Read the model definition and answer for the solid it produces. Units are mm, in the model's axes. Coordinates: 2 decimals unless noted, no trailing zeros. Loops run counter-clockwise (first coordinate to the right, second up) from the corner with the lowest first, then second, coordinate; pieces in that order, holes last.
Q1. Straight lines are drawn through the part: line 1 (X direction, y = 5.1, z = 127.5); line 2 (X direction, y = 0.55, z = 251); line 3 (Y direction, x = 12, z = 236.5). For each, find the intervals that lie inside material, in ascending order.
Q2. Section A-A (z = 50) is taken. Give the vertices of the cut face in (x, y), then the cut area to 3 significant figures.
Q3. Section B-B (y = 3.65) is taken. Give the vertices of the cut face in (x, z).
Q4. Flat-ended cylindrical pins translate along their axes: P1, Ø1.5, axis at y = 2.5, z = 259.5, coming from the +X side; P2, Ø1.1, axis at x = -19, y = 0.5, coming from the +Z side; P3, Ø4, axis at x = -20.5, z = 234.5, coming from the +Y side. Find the tip coordinate at first contact, or state that the pin passes through.
Q5. Section C-C (x = 2) is taken. Count the separate pieces of the cut face and the enclosed holes in it, then the cut area to 3 significant figures.
from build123d import *

# Parameters (mm, degrees)
BOSS_EXTRUDE1_DEPTH   = 320
BOSS_EXTRUDE1_2_DEPTH = 320
SKETCH3_W             = 45
SKETCH3_H             = 6
BOSS_EXTRUDE2_DEPTH   = 1


with BuildPart() as part:
    # Sketch1 → Boss-Extrude1 (new body)
    with BuildSketch(Plane.XY):
        Polygon((-17.5, 0), (-17.5, 6), (-15.5, 6), (-15.5, 1), (-11.5, 1), (-11.5, 0), align=None)
    extrude(amount=BOSS_EXTRUDE1_DEPTH)



with BuildPart() as body_2:
    # Sketch1 → Boss-Extrude1 2 (new body)
    with BuildSketch(Plane.XY):
        Polygon((17.5, 0), (17.5, 6), (15.5, 6), (15.5, 1), (11.5, 1), (11.5, 0), align=None)
    extrude(amount=BOSS_EXTRUDE1_2_DEPTH)


with BuildPart() as part_1:
    add(part.part)

    add(body_2.part)  # Boss-Extrude2 merges body 2
    # Sketch3 → Boss-Extrude2 (add)
    with BuildSketch(Plane(origin=(0, 0, 0), x_dir=(1, 0, 0), z_dir=(0, 1, 0))):
        with Locations((0, -14)):
            Rectangle(SKETCH3_W, SKETCH3_H)
        with Locations((0, -36)):
            Rectangle(SKETCH3_W, SKETCH3_H)
        with Locations((0, -58)):
            Rectangle(SKETCH3_W, SKETCH3_H)
        with Locations((0, -80)):
            Rectangle(SKETCH3_W, SKETCH3_H)
        with Locations((0, -102)):
            Rectangle(SKETCH3_W, SKETCH3_H)
        with Locations((0, -124)):
            Rectangle(SKETCH3_W, SKETCH3_H)
        with Locations((0, -146)):
            Rectangle(SKETCH3_W, SKETCH3_H)
        with Locations((0, -168)):
            Rectangle(SKETCH3_W, SKETCH3_H)
        with Locations((0, -190)):
            Rectangle(SKETCH3_W, SKETCH3_H)
        with Locations((0, -212)):
            Rectangle(SKETCH3_W, SKETCH3_H)
        with Locations((0, -234)):
            Rectangle(SKETCH3_W, SKETCH3_H)
        with Locations((0, -256)):
            Rectangle(SKETCH3_W, SKETCH3_H)
        with Locations((0, -278)):
            Rectangle(SKETCH3_W, SKETCH3_H)
        with Locations((0, -300)):
            Rectangle(SKETCH3_W, SKETCH3_H)
    extrude(amount=BOSS_EXTRUDE2_DEPTH)


solid = part_1.part
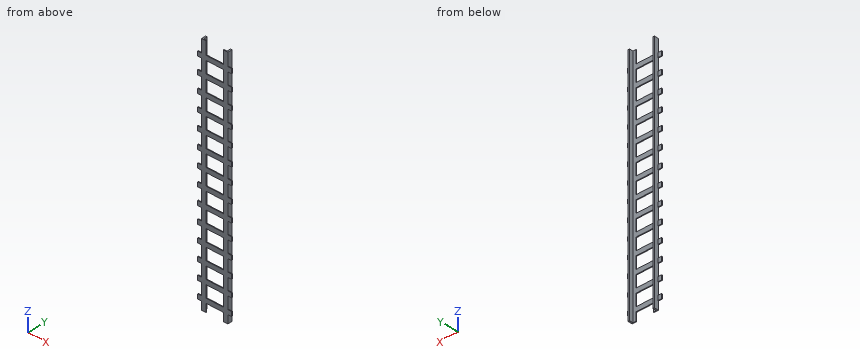
Numbers:
1. line 1: x = -17.5 to -15.5, 15.5 to 17.5
1. line 2: x = -17.5 to -11.5, 11.5 to 17.5
1. line 3: y = 0 to 1
2. outline: (-17.5, 0) - (-11.5, 0) - (-11.5, 1) - (-15.5, 1) - (-15.5, 6) - (-17.5, 6) - close; (11.5, 0) - (17.5, 0) - (17.5, 6) - (15.5, 6) - (15.5, 1) - (11.5, 1) - close
2. area: 32.0 mm2
3. outline: (-17.5, 0) - (-15.5, 0) - (-15.5, 320) - (-17.5, 320) - close; (15.5, 0) - (17.5, 0) - (17.5, 320) - (15.5, 320) - close
4. P1: stops at x = 17.5
4. P2: stops at z = 303
4. P3: stops at y = 1
5. separate pieces: 14
5. enclosed holes: 0
5. area: 84.0 mm2
